```python
from build123d import *

# Parameters (mm, degrees)
F0_R     = 10.16
F1_DEPTH = 15.7734
F2_DEPTH = 40.2336


with BuildPart() as f1:
    # F0 (on Top) → F1 (new body)
    with BuildSketch(Plane.XY):
        with BuildLine():
            Line((57.792583, 18.78227), (9.413565, 26.979908))
            ThreePointArc((9.413565, 26.979908), (23.297245, 16.545967), (28.575, 0))
            ThreePointArc((28.575, 0), (23.297245, -16.545967), (9.413565, -26.979908))
            Line((9.413565, -26.979908), (57.792583, -18.78227))
            ThreePointArc((57.792583, -18.78227), (73.66, 0), (57.792583, 18.78227))
        make_face()
        with Locations((54.61, 0)):
            Circle(F0_R, mode=Mode.SUBTRACT)
    extrude(amount=F1_DEPTH)

    # F0 (on Top) → F2 (join)
    with BuildSketch(Plane.XY):
        with BuildLine():
            Line((9.413565, 26.979908), (0, 28.575))
            ThreePointArc((0, 28.575), (-28.575, 0), (0, -28.575))
            Line((0, -28.575), (9.413565, -26.979908))
            ThreePointArc((9.413565, -26.979908), (23.297245, -16.545967), (28.575, 0))
            ThreePointArc((28.575, 0), (23.297245, 16.545967), (9.413565, 26.979908))
        make_face()
        with BuildLine():
            ThreePointArc((13.447765, -4.826), (-14.2875, 0), (13.447765, 4.826))
            Line((13.447765, 4.826), (18.5293, 4.826))
            Line((18.5293, 4.826), (18.5293, -4.826))
            Line((18.5293, -4.826), (13.447765, -4.826))
        make_face(mode=Mode.SUBTRACT)
    extrude(amount=F2_DEPTH)


solid = f1.part
```
Geometry check sheet. Reference: the model listing, model coordinates, mm. A direction names the side the tool comes from. Give positions to 0.01 mm unless a question says otherwise; leave off trailing zeros. Write each loop counter-clockwise with the first axis right and the second up, starting at its lowest first coordinate (ties: lowest second). Pieces come first, ordered by that corner, then holes. Notation, with made-up numbers: (20, -19) -> (76, -19) arc R18 cw to (76, -3) -> close; hole circle Ø2 at (79, 45). An arc over 180 degrees is marked (long way). Use one line per item in the form item = value.
Item 1: Depth check by flat-ended pin: pin 1 Ø5 at (y, z) = (0, 25.5) entering from -X (3 decimals); pin 2 Ø1 at (x, z) = (42.5, 14) entering from +Y; pin 3 Ø12 at (x, y) = (49, -2.5) entering from +Z; pin 4 Ø12 at (x, y) = (59, 13.5) entering from -Z. Enter the tip coordinate at first touch or a pass-through.
Results list:
pin_1 = -28.575
pin_2 = 21.46
pin_3 = 15.77
pin_4 = 0
Item 2: Sectioned sample at B-B on x = 54.61. Enter the section's corners in (y, z).
Results list:
outline = (-19.32, 0) -> (-10.16, 0) -> (-10.16, 15.77) -> (-19.32, 15.77) -> close; (10.16, 0) -> (19.32, 0) -> (19.32, 15.77) -> (10.16, 15.77) -> close
Item 3: Access from +Z, -Z, +X, -X, +Y, -Y to the whole of each face (thin tool, end or side, straight path). Record for faces 4 (the flat face through (22, 0, 0)), 5 (the flat face through (16, 4.826, 20)).
Results list:
face_4 = -Z, +X, -X, +Y, -Y
face_5 = +Z, -Z
Item 4: Sectioned sample at C-C on y = -1. Enter the section's corners in (x, z), plus the area to 3 significant figures.
Results list:
outline = (-28.56, 0) -> (-14.25, 0) -> (-14.25, 40.23) -> (-28.56, 40.23) -> close; (18.53, 0) -> (44.5, 0) -> (44.5, 15.77) -> (28.56, 15.77) -> (28.56, 40.23) -> (18.53, 40.23) -> close; (64.72, 0) -> (73.63, 0) -> (73.63, 15.77) -> (64.72, 15.77) -> close
area = 1,370 mm2
Item 5: Sectioned sample at D-D on x = -1.5. Enter the section's corners in (y, z), plus the area to 3 significant figures.
Results list:
outline = (-28.54, 0) -> (-14.21, 0) -> (-14.21, 40.23) -> (-28.54, 40.23) -> close; (14.21, 0) -> (28.54, 0) -> (28.54, 40.23) -> (14.21, 40.23) -> close
area = 1,150 mm2
Item 6: Scan lines: line 1 (X direction, y = 0, z = 19) (1 decimal); line 2 (Y direction, x = -4, z = 5.5); line 3 (Y direction, x = 17, z = 24). Record each from-to range of solid material in increasing order.
Results list:
line_1 = -28.6 to -14.3, 18.5 to 28.6
line_2 = -28.29 to -13.72, 13.72 to 28.29
line_3 = -22.97 to -4.83, 4.83 to 22.97
Item 7: Mould release check, pull along Y, two halves, no side actions. Record for faces 1 (the flat face through (18.529, 0, 20)), 2 (the cylindrical face through (73.656, -0.374, 7.776)), 3 (the flat face through (41, 0, 15.773)): released by +Y, released by -Y, zero draft, split by the parting line, or undercut.
Results list:
face_1 = undercut
face_2 = split by the parting line
face_3 = zero draft
